Check sheet for the modelled part. Datum: model origin and axes. Units: mm. Face numbers are marked on the shaded views. A direction names the side the tool comes from. Coordinates: 2 decimals unless noted, no trailing zeros. Write each loop counter-clockwise with the first axis right and the second up, starting at its lowest first coordinate (ties: lowest second). Pieces come first, ordered by that corner, then holes. Notation, with made-up numbers: (-7, -16) -> (49, -16) arc R24 ccw to (49, 0) -> close; hole circle Ø5 at (29.25, 58.5). An arc over 180 degrees is marked (long way). One line per item, written item: value. Start each with the question number.
1) Scan lines: line 1 along Z through (x, y) = (26, -3.6); line 2 along Z through (x, y) = (-43.18, -1.9) (3 decimals); line 3 along Z through (x, y) = (25.5, -2.7). Record each from-to range of solid material in increasing order. Write a range as [from, to].
2) Sectioned sample at B-B on z = 38.1. Enter the section's corners in (x, y) (3 decimals).
3) Sectioned sample at A-A on y = -1.5. Give the number of separate pieces and of enclosed holes in the cut face, plus the area to 3 significant figures.
4) Set-up check for the marked faces 3 and 4: record each of +Z, -Z, +X, -X, +Y, -Y from which the full face is reachable in a straight line by a thin tool's end or side.
5) Draft check along X on the marked faces 1 and 2. Enter one of: +X half, -X half, draft (parallel to the pull), parting line (faces both ways), or undercut.
6) Sectioned sample at D-D on x = 0. Enter the section's corners in (y, z), plus the area to 3 significant figures.
7) Sectioned sample at C-C on x = -43.18. Enter the section's corners in (y, z) (3 decimals).
8) Gauge pin test, flat end, axial feed: P1, Ø1, axis at x = 29, z = -10.5, coming from the -Y side. Record the tip position at first contact, or that the pin passes through.
```python
from build123d import *

# Parameters (mm, degrees)
F0_W      = 101.6
F0_H      = 101.6
F1_DEPTH  = 5.08
F3_D      = 6.35
F5_DEPTH  = 2.54
F6_R      = 5.08
F7_R      = 1.27
F9_DEPTH  = 2.54
F10_R     = 5.08
F11_R     = 1.27
F12_R     = 5
F13_DEPTH = 25
F14_SIZE  = 0.2
F15_SIZE  = 5


with BuildPart() as f1:
    # F0 (on Front) → F1 (new body)
    with BuildSketch(Plane.XZ):
        Rectangle(F0_W, F0_H)
    extrude(amount=F1_DEPTH)

    # F3 (through all)
    with Locations(Plane(origin=(0, 0, 0), x_dir=(1, 0, 0), z_dir=(0, 1, 0))):
        with Locations((-43.18, 38.1), (-43.18, 19.05), (-43.18, 0), (-43.18, -19.05), (-43.18, -38.1)):
            Hole(F3_D / 2)

    # F4 (on face) → F5 (cut)
    with BuildSketch(Plane.XZ.offset(5.08)):
        with BuildLine():
            Line((-19.9187304825, 34.667711705), (-19.9187304825, -34.667711705))
            Line((-19.9187304825, -34.667711705), (19.9187304825, -34.667711705))
            Line((19.9187304825, -34.667711705), (19.9187304825, -24.3936947418))
            ThreePointArc((19.9187304825, -24.3936947418), (5.4860749886, 0), (19.9187304825, 24.3936947418))
            Line((19.9187304825, 24.3936947418), (19.9187304825, 34.667711705))
            Line((19.9187304825, 34.667711705), (-19.9187304825, 34.667711705))
        make_face()
    extrude(amount=-F5_DEPTH, mode=Mode.SUBTRACT)

    # F6
    f6_edges = [f1.edges().sort_by_distance(p)[0] for p in [
        (-19.91873, -3.81, 34.667712),
        (19.91873, -3.81, 34.667712),
        (19.91873, -3.81, 24.393695),
        (19.91873, -3.81, -24.393695),
        (19.91873, -3.81, -34.667712),
        (-19.91873, -3.81, -34.667712),
    ]]
    fillet(f6_edges, radius=F6_R)

    # F7
    f7_edges = [f1.edges().sort_by_distance(p)[0] for p in [
        (19.91873, -2.54, 28.410832),
        (19.327372, -2.54, 24.855192),
        (18.430833, -2.54, 33.179814),
        (5.486075, -2.54, 0),
        (0, -2.54, 34.667712),
        (19.327372, -2.54, -24.855192),
        (-18.430833, -2.54, 33.179814),
        (19.91873, -2.54, -28.410832),
        (-19.91873, -2.54, 0),
        (18.430833, -2.54, -33.179814),
        (-18.430833, -2.54, -33.179814),
        (0, -2.54, -34.667712),
    ]]
    fillet(f7_edges, radius=F7_R)

    # F8 (on face) → F9 (cut)
    with BuildSketch(Plane.XZ.offset(5.08)):
        with BuildLine():
            Line((38.1, 19.05), (22.8523529701, 19.05))
            ThreePointArc((22.8523529701, 19.05), (11.5820746869, 0), (22.8523529701, -19.05))
            Line((22.8523529701, -19.05), (38.1, -19.05))
            Line((38.1, -19.05), (38.1, 19.05))
        make_face()
    extrude(amount=-F9_DEPTH, mode=Mode.SUBTRACT)

    # F10
    f10_edges = [f1.edges().sort_by_distance(p)[0] for p in [
        (22.852353, -3.81, 19.05),
        (38.1, -3.81, 19.05),
        (38.1, -3.81, -19.05),
        (22.852353, -3.81, -19.05),
    ]]
    fillet(f10_edges, radius=F10_R)

    # F11
    f11_edges = [f1.edges().sort_by_distance(p)[0] for p in [
        (28.634501, -2.54, -19.05),
        (22.8067, -2.54, -18.840951),
        (36.612102, -2.54, -17.562102),
        (11.582075, -2.54, 0),
        (38.1, -2.54, 0),
        (22.8067, -2.54, 18.840951),
        (36.612102, -2.54, 17.562102),
        (28.634501, -2.54, 19.05),
    ]]
    fillet(f11_edges, radius=F11_R)

    # F12 (on face) → F13 (cut)
    with BuildSketch(Plane.XZ.offset(5.08)):
        with Locations((28.6345014435, 30)):
            Circle(F12_R)
        with Locations((28.6345014435, -30)):
            Circle(F12_R)
    extrude(amount=-F13_DEPTH, mode=Mode.SUBTRACT)

    # F14
    f14_edges = [f1.edges().sort_by_distance(p)[0] for p in [
        (23.634501, -5.08, 30),
        (23.634501, -5.08, -30),
        (33.634501, -2.54, -30),
        (23.634501, 0, -30),
    ]]
    chamfer(f14_edges, length=F14_SIZE)

    # F15
    f15_edges = [f1.edges().sort_by_distance(p)[0] for p in [
        (50.8, -2.54, -50.8),
        (50.8, -2.54, 50.8),
        (-50.8, -2.54, -50.8),
        (-50.8, -2.54, 50.8),
    ]]
    chamfer(f15_edges, length=F15_SIZE)


solid = f1.part
```
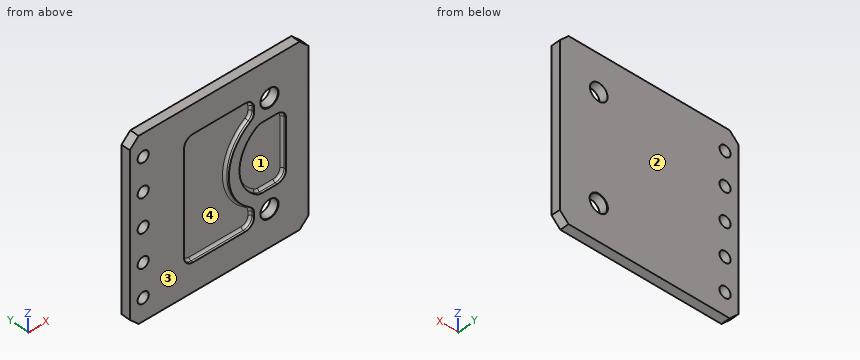
Answers:
1. line 1: z = [-50.8, -34.25], [-25.75, -19.03], [19.03, 25.75], [34.25, 50.8]
1. line 2: z = [-50.8, -41.275], [-34.925, -22.225], [-15.875, -3.175], [3.175, 15.875], [22.225, 34.925], [41.275, 50.8]
1. line 3: z = [-50.8, -33.9], [-26.1, -18.4], [18.4, 26.1], [33.9, 50.8]
2. outline: (-50.8, -5.08) -> (-46.355, -5.08) -> (-46.355, 0) -> (-50.8, 0) -> close; (-40.005, -5.08) -> (50.8, -5.08) -> (50.8, 0) -> (-40.005, 0) -> close
3. separate pieces: 1
3. enclosed holes: 7
3. area: 9,960 mm2
4. face 3: +Z, -Z, +X, -X, -Y
4. face 4: -Y
5. face 1: undercut
5. face 2: draft
6. outline: (-5.08, -50.8) -> (0, -50.8) -> (0, 50.8) -> (-5.08, 50.8) -> (-5.08, 34.67) -> (-3.81, 34.67) arc R1.27 cw to (-2.54, 33.4) -> (-2.54, -33.4) arc R1.27 cw to (-3.81, -34.67) -> (-5.08, -34.67) -> close
6. area: 341 mm2
7. outline: (-5.08, -50.8) -> (0, -50.8) -> (0, -41.275) -> (-5.08, -41.275) -> close; (-5.08, -34.925) -> (0, -34.925) -> (0, -22.225) -> (-5.08, -22.225) -> close; (-5.08, -15.875) -> (0, -15.875) -> (0, -3.175) -> (-5.08, -3.175) -> close; (-5.08, 3.175) -> (0, 3.175) -> (0, 15.875) -> (-5.08, 15.875) -> close; (-5.08, 22.225) -> (0, 22.225) -> (0, 34.925) -> (-5.08, 34.925) -> close; (-5.08, 41.275) -> (0, 41.275) -> (0, 50.8) -> (-5.08, 50.8) -> close
8. P1: stops at y = -2.54
